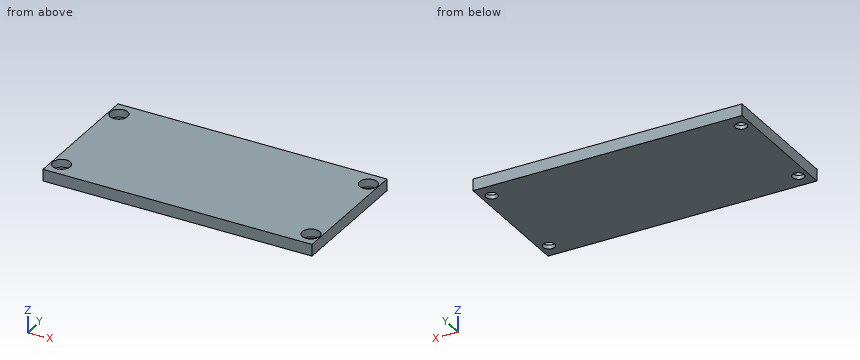
```python
from build123d import *

# Parameters (mm, degrees)
SZKIC1_W                    = 69
SZKIC1_H                    = 34
DODANIE_WYCI_GNI_CIE1_DEPTH = 3
SZKIC2_R                    = 1.5
WYTNIJ_WYCI_GNI_CIE1_DEPTH  = 3
SZKIC3_R                    = 2.25
WYTNIJ_WYCI_GNI_CIE2_DEPTH  = 2


with BuildPart() as part:
    # Szkic1 → Dodanie-wyciągnięcie1 (new body)
    with BuildSketch(Plane.XY):
        with Locations((34.5, 17)):
            Rectangle(SZKIC1_W, SZKIC1_H)
    extrude(amount=DODANIE_WYCI_GNI_CIE1_DEPTH)

    # Szkic2 → Wytnij-wyciągnięcie1 (cut)
    with BuildSketch(Plane.XY.offset(3)):
        with Locations((2.5, 30)):
            Circle(SZKIC2_R)
        with Locations((2.5, 4)):
            Circle(SZKIC2_R)
        with Locations((66.5, 4)):
            Circle(SZKIC2_R)
        with Locations((66.5, 30)):
            Circle(SZKIC2_R)
    extrude(amount=-WYTNIJ_WYCI_GNI_CIE1_DEPTH, mode=Mode.SUBTRACT)

    # Szkic3 → Wytnij-wyciągnięcie2 (cut)
    with BuildSketch(Plane.XY.offset(3)):
        with Locations((2.5, 30)):
            Circle(SZKIC3_R)
        with Locations((66.5, 30)):
            Circle(SZKIC3_R)
        with Locations((2.5, 4)):
            Circle(SZKIC3_R)
        with Locations((66.5, 4)):
            Circle(SZKIC3_R)
    extrude(amount=-WYTNIJ_WYCI_GNI_CIE2_DEPTH, mode=Mode.SUBTRACT)


solid = part.part
```
Can you work these out from the model? Positions are in its coordinate system, mm. Round coordinates to 2 decimals unless told otherwise and drop trailing zeros. Order: outer loops, then holes, each group sorted by start corner. A loop starts at its lowest first (then second) coordinate and runs counter-clockwise, first axis right, second up. Notation, with made-up numbers: (47, 77) -> (64, 77) arc R17 ccw to (64, 98) -> close; hole circle Ø7 at (6, 74.5). An arc over 180 degrees is marked (long way). Return JSON: item names as keys, results as strings. Group by question number.
1. I need wall thicknesses on line 1 (Y direction, x = 66.5, z = 1.9); line 2 (X direction, y = 28, z = 2.8); line 3 (X direction, y = 29, z = 1.65). Which ranges of each line are inside material? Lowest first, please. Write a range as [from, to].
2. If we section it at C-C, the plane z = 2.2: Write out the boundary of the cut face in (x, y), then the cut area to 3 significant figures.
3. If we section it at A-A, the plane x = 66.5: Write out the boundary of the cut face in (y, z), then the cut area to 3 significant figures.
4. Will these pins go through, and if not, where does the flat tip stop? pin 1 (6 mm diameter, centred on x = 2.5, y = 30, fed in from -Z); pin 2 (2 mm diameter, centred on x = 67, y = 4.5, fed in from +Z); pin 3 (2.5 mm diameter, centred on x = 2.5, y = 30, fed in from -Z).
5. If we section it at B-B, the plane y = 30: Write out the boundary of the cut face in (x, z), then the cut area to 3 significant figures.
Output values:
{
 "1": {"line 1": "[0, 1.75], [6.25, 27.75], [32.25, 34]", "line 2": "[0, 1.47], [3.53, 65.47], [67.53, 69]", "line 3": "[0, 0.48], [4.52, 64.48], [68.52, 69]"},
 "2": {"outline": "(0, 0) -> (69, 0) -> (69, 34) -> (0, 34) -> close; hole circle Ø4.5 at (2.5, 4); hole circle Ø4.5 at (2.5, 30); hole circle Ø4.5 at (66.5, 4); hole circle Ø4.5 at (66.5, 30)", "area": "2,280 mm²"},
 "3": {"outline": "(0, 0) -> (2.5, 0) -> (2.5, 1) -> (1.75, 1) -> (1.75, 3) -> (0, 3) -> close; (5.5, 0) -> (28.5, 0) -> (28.5, 1) -> (27.75, 1) -> (27.75, 3) -> (6.25, 3) -> (6.25, 1) -> (5.5, 1) -> close; (31.5, 0) -> (34, 0) -> (34, 3) -> (32.25, 3) -> (32.25, 1) -> (31.5, 1) -> close", "area": "78.0 mm²"},
 "4": {"pin 1": "z = 0", "pin 2": "z = 1", "pin 3": "through"},
 "5": {"outline": "(0, 0) -> (1, 0) -> (1, 1) -> (0.25, 1) -> (0.25, 3) -> (0, 3) -> close; (4, 0) -> (65, 0) -> (65, 1) -> (64.25, 1) -> (64.25, 3) -> (4.75, 3) -> (4.75, 1) -> (4, 1) -> close; (68, 0) -> (69, 0) -> (69, 3) -> (68.75, 3) -> (68.75, 1) -> (68, 1) -> close", "area": "183 mm²"}
}
